Source: CAD feature listing. Evaluate the final solid. Frame: model axes, mm. A direction names the side the tool comes from. Round coordinates to 2 decimals unless told otherwise and drop trailing zeros. Loops run counter-clockwise (first coordinate to the right, second up) from the corner with the lowest first, then second, coordinate; pieces in that order, holes last.
Item 1: Ray query, L1, parallel to X at y = 22, z = -2.5; L2, parallel to X at y = 10, z = 75; L3, parallel to X at y = 12, z = 36. Return the intervals inside material, ascending.
Item 2: Section query C-C on x = -122. Return loops of the section in (y, z).
Item 3: Section query D-D on x = -84. Return loops of the section in (y, z).
Item 4: First-contact query: P1, Ø10, axis at y = 19, z = 13.5, coming from the -X side; P2, Ø5, axis at x = -81.5, y = 11.5, coming from the +Z side; P3, Ø12, axis at x = -95.5, y = 16, coming from the -Z side. Flat tips, straight axial feed; report the tip coordinate or a pass-through.
Item 5: Section query B-B on z = 111.5. Return loops of the section in (x, y), then the cut area to 3 significant figures.
Item 6: Access query for faces 1 (the cylindrical face through (-36.707, 8.217, 74.001)), 2 (the flat face through (-16, 16.667, 65)), 3 (the flat face through (162.5, 12, -2)). Directions: +Z, -Z, +X, -X, +Y, -Y. A direction counts if a zero-diameter tool reaches every point of the face in a straight line with its end or side. Return the directions, or none.
Item 7: Section query A-A on y = 7.5. Return loops of the section in (x, z), then the cut area to 3 significant figures.
```python
from build123d import *

# Parameters (mm, degrees)
F3_DEPTH = 25
F4_DEPTH = 16.6666666667
F5_W     = 25
F5_H     = 300
F6_DEPTH = 400


with BuildPart() as f3:
    # F2 (on Front) → F3 (new body)
    with BuildSketch(Plane.XZ):
        with BuildLine():
            Line((162.5, 150), (-12.5, 150))
            ThreePointArc((-12.5, 150), (13.6340385875, 77.0146090037), (22.5, 0))
            ThreePointArc((22.5, 0), (0, -22.5), (-22.5, 0))
            ThreePointArc((-22.5, 0), (-36.3223137223, 73.0281778836), (-75.877047, 135.9534843745))
            ThreePointArc((-75.877047, 135.9534843745), (-139.0040652509, 80.6022423696), (-162.5, 0))
            ThreePointArc((-162.5, 0), (-118.566017178, -106.066017178), (-12.5, -150))
            Line((-12.5, -150), (162.5, -150))
            Line((162.5, -150), (162.5, 150))
        make_face()
        with BuildLine():
            ThreePointArc((22.5, 0), (13.6340385875, 77.0146090037), (-12.5, 150))
            ThreePointArc((-12.5, 150), (-44.9574902282, 146.4462745449), (-75.877047, 135.9534843745))
            ThreePointArc((-75.877047, 135.9534843745), (-36.3223137223, 73.0281778836), (-22.5, 0))
            ThreePointArc((-22.5, 0), (0, -22.5), (22.5, 0))
        make_face()
    extrude(amount=-F3_DEPTH)

    # F2 (on Front) → F4 (cut)
    with BuildSketch(Plane.XZ):
        with BuildLine():
            ThreePointArc((22.5, 0), (13.6340385875, 77.0146090037), (-12.5, 150))
            ThreePointArc((-12.5, 150), (-44.9574902282, 146.4462745449), (-75.877047, 135.9534843745))
            ThreePointArc((-75.877047, 135.9534843745), (-36.3223137223, 73.0281778836), (-22.5, 0))
            ThreePointArc((-22.5, 0), (0, -22.5), (22.5, 0))
        make_face()
    extrude(amount=-F4_DEPTH, mode=Mode.SUBTRACT)


with BuildPart() as f6:
    # F5 (on face) → F6 (new body)
    with BuildSketch(Plane(origin=(0, 25, 0), x_dir=(-1, 0, 0), z_dir=(0, 1, 0))):
        with Locations((-150, 0)):
            Rectangle(F5_W, F5_H)
    extrude(amount=-F6_DEPTH)


with BuildPart() as f9_1:
    # F9: instance of F3
    add(f3.part.mirror(Plane(origin=(150, -175, 0), x_dir=(-1, 0, 0), z_dir=(0, -1, 0))))


with BuildPart() as f10_1:
    # F10: copy of F3
    add(f3.part)


solid = f3.part
```
Data:
1. L1: x = -162.48 to 162.5
1. L2: x = -142.4 to -37.11, 14.1 to 162.5
1. L3: x = -158.12 to -25.77, 20.58 to 162.5
2. outline: (0, -102.52) - (25, -102.52) - (25, 102.52) - (0, 102.52) - close
3. outline: (0, -131.86) - (25, -131.86) - (25, 131.86) - (0, 131.86) - close
4. P1: stops at x = -162.26
4. P2: stops at z = 134.45
4. P3: stops at z = -128.73
5. outline: (-112.84, 0) - (-56.5, 0) - (-56.5, 16.67) - (3.63, 16.67) - (3.63, 0) - (162.5, 0) - (162.5, 25) - (-112.84, 25) - close
5. area: 5,880 mm2
6. face 1: +Z, -Y
6. face 2: -Y
6. face 3: +Z, -Z, +X, +Y, -Y
7. outline: (-75.88, 135.95) arc R150 ccw to (-12.5, -150) - (162.5, -150) - (162.5, 150) - (-12.5, 150) arc R338.93 cw to (22.5, 0) arc R22.5 cw to (-22.5, 0) arc R199.83 ccw to start
7. area: 79,300 mm2
